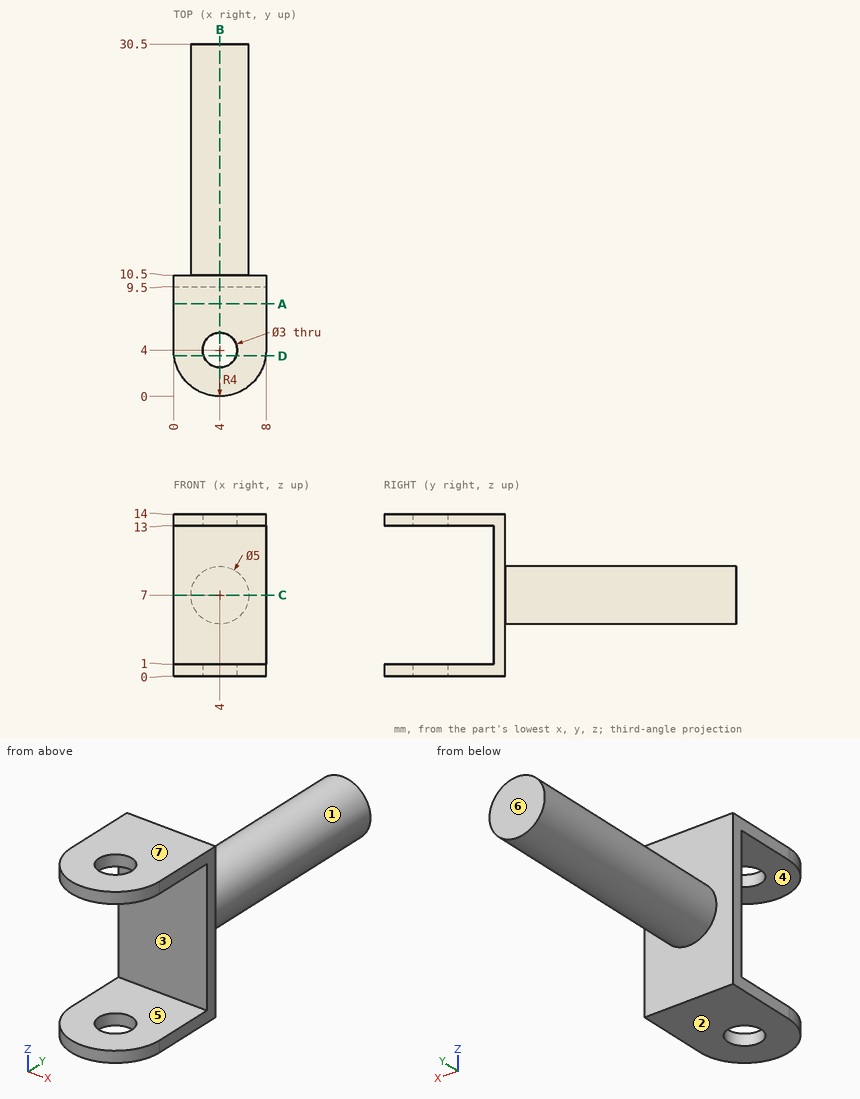
Geometry check sheet. Reference: drawing and pictorial views, mm from the part's lowest x, y, z. A direction names the side the tool comes from. Give positions to 0.01 mm unless a question says otherwise; leave off trailing zeros. Order: outer loops, then holes, each group sorted by start corner. A loop starts at its lowest first (then second) coordinate and runs counter-clockwise, first axis right, second up. Notation, with made-up numbers: M -34,50.25 L 22,50.25 A18 ccw 22,61.25 Z; hole C -2,6.25 d7. An arc over 180 degrees is marked long. Use one line per item in the form item = value. Start each with the question number.
Q1. Section check D-D (y = 3.5). Enter the section's corners in (x, z), then the cut area to 3 significant figures.
Q2. Access from +Z, -Z, +X, -X, +Y, -Y to the whole of each face (thin tool, end or side, straight path). Record for the marked faces 1, 2 and 3.
Q3. Section check C-C (z = 7). Enter the section's corners in (x, y).
Q4. Section check A-A (y = 8). Enter the section's corners in (x, z), then the cut area to 3 significant figures.
Q5. Section check B-B (x = 4). Enter the section's corners in (y, z), then the cut area to 3 significant figures.
Q6. Scan lines: line 1 along Z through (x, y) = (3, 1); line 2 along Y through (x, z) = (4, 0.3); line 3 along X through (y, z) = (4, 0.5). Record each from-to range of solid material in increasing order. Write a range as [from, to].
Q7. Go/stop test with flat-tipped pins: pin 1 Ø2 at (x, z) = (2, 2.5) entering from +Y; pin 2 Ø3 at (x, y) = (2, 21.5) entering from +Z; pin 3 Ø1 at (y, z) = (11.5, 8) entering from -X. Record where each tip stops, or that it passes through.
Q8. Mould release check, pull along Z, two halves, no side actions. Record for the marked faces 4, 5, 6 and 7: +Z half, -Z half, draft (parallel to the pull), parting line (faces both ways), or undercut.
Evaluation:
q1.outline = M 0.03,0 L 2.59,0 L 2.59,1 L 0.03,1 Z; M 0.03,13 L 2.59,13 L 2.59,14 L 0.03,14 Z; M 5.41,0 L 7.97,0 L 7.97,1 L 5.41,1 Z; M 5.41,13 L 7.97,13 L 7.97,14 L 5.41,14 Z
q1.area = 10.2 mm2
q2.face_1 = +Y
q2.face_2 = -Z, +X, -X, +Y, -Y
q2.face_3 = +X, -X, -Y
q3.outline = M 0,9.5 L 8,9.5 L 8,10.5 L 6.5,10.5 L 6.5,30.5 L 1.5,30.5 L 1.5,10.5 L 0,10.5 Z
q4.outline = M 0,0 L 8,0 L 8,1 L 0,1 Z; M 0,13 L 8,13 L 8,14 L 0,14 Z
q4.area = 16.0 mm2
q5.outline = M 0,0 L 2.5,0 L 2.5,1 L 0,1 Z; M 0,13 L 2.5,13 L 2.5,14 L 0,14 Z; M 5.5,0 L 10.5,0 L 10.5,4.5 L 30.5,4.5 L 30.5,9.5 L 10.5,9.5 L 10.5,14 L 5.5,14 L 5.5,13 L 9.5,13 L 9.5,1 L 5.5,1 Z
q5.area = 127 mm2
q6.line_1 = [0, 1], [13, 14]
q6.line_2 = [0, 2.5], [5.5, 10.5]
q6.line_3 = [0, 2.5], [5.5, 8]
q7.pin_1 = 10.5
q7.pin_2 = 9.45
q7.pin_3 = 1.55
q8.face_4 = undercut
q8.face_5 = undercut
q8.face_6 = draft
q8.face_7 = +Z half
